Geometry check sheet. Reference: the model listing, model coordinates, mm. Round coordinates to 2 decimals unless told otherwise and drop trailing zeros. Write each loop counter-clockwise with the first axis right and the second up, starting at its lowest first coordinate (ties: lowest second). Pieces come first, ordered by that corner, then holes. Notation, with made-up numbers: M 75,63 L 85,63 A35 ccw 85,101 Z; hole C 51,58.25 d3. An arc over 180 degrees is marked long. Answer as CSV lines item,"result". Start each with the question number.
```python
from build123d import *

# Parameters (mm, degrees)
PROFILE_DEPTH     = 419.1
MITER1_DEPTH      = 422.259210582
MITER1_DEPTH_BACK = 422.259210582
MITER2_DEPTH      = 422.259210582
MITER2_DEPTH_BACK = 422.259210582


with BuildPart() as part:
    # Sketch1 → Profile (new body)
    with BuildSketch(Plane.XY):
        Polygon((-19.05, -38.1), (-4, -38.1), (-4, -30.1), (4, -30.1), (4, -38.1), (19.05, -38.1), (19.05, -23.05), (11.05, -23.05), (11.05, -15.05), (19.05, -15.05), (19.05, 15.05), (11.05, 15.05), (11.05, 23.05), (19.05, 23.05), (19.05, 38.1), (4, 38.1), (4, 30.1), (-4, 30.1), (-4, 38.1), (-19.05, 38.1), (-19.05, 23.05), (-11.05, 23.05), (-11.05, 15.05), (-19.05, 15.05), (-19.05, -15.05), (-11.05, -15.05), (-11.05, -23.05), (-19.05, -23.05), align=None)
    extrude(amount=PROFILE_DEPTH)

    # Sketch2 → Miter1 (cut, two sides: drawn at the far end of the back side and taken through both)
    with BuildSketch(Plane(origin=(0, 0, 0), x_dir=(1, 0, 0), z_dir=(0, 1, 0)).offset(-MITER1_DEPTH_BACK)):
        Polygon((-19.05, -419.1), (25, -342.8), (25, -430), align=None)
    extrude(amount=MITER1_DEPTH + MITER1_DEPTH_BACK, mode=Mode.SUBTRACT)

    # Sketch3 → Miter2 (cut, two sides: drawn at the far end of the back side and taken through both)
    with BuildSketch(Plane(origin=(0, 0, 0), x_dir=(1, 0, 0), z_dir=(0, 1, 0)).offset(-MITER2_DEPTH_BACK)):
        Polygon((-19.05, 0), (25, 10), (25, -25.43), align=None)
    extrude(amount=MITER2_DEPTH + MITER2_DEPTH_BACK, mode=Mode.SUBTRACT)


solid = part.part
```
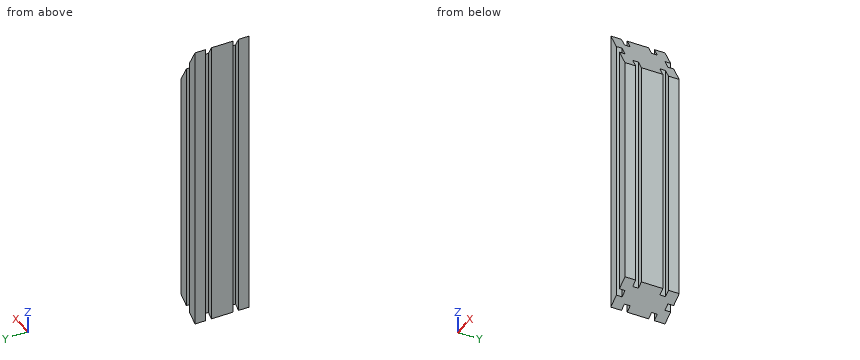
1) Section check B-B, the plane z = 81.5. Record the cut outline in (x, y).
2) Scan lines: line 1 (Y direction, x = -16.5, z = 248); line 2 (X direction, y = 21.5, z = 21.5); line 3 (Y direction, x = 2.5, z = 278). Record each from-to range of solid material in increasing order. Write a range as from..to.
3) Section check A-A, the plane x = 15.5. Record the cut outline in (y, z).
4) Go/stop test with flat-tipped pins: pin 1 (10 mm diameter, centred on x = 1.5, y = 23.5, fed in from -Z); pin 2 (1 mm diameter, centred on x = -2.5, z = 341, fed in from -Y); pin 3 (12 mm diameter, centred on y = -29.5, z = 370, fed in from +X). Record where each tip stops, or that it passes through.
5) Section check D-D, the plane y = 19.5. Record the cut outline in (x, z), plus the area to 3 significant figures.
6) Section check C-C, the plane y = 3. Record the cut outline in (x, z), plus the area to 3 significant figures.
Results:
1,outline,"M -19.05,-38.1 L -4,-38.1 L -4,-30.1 L 4,-30.1 L 4,-38.1 L 19.05,-38.1 L 19.05,-23.05 L 11.05,-23.05 L 11.05,-15.05 L 19.05,-15.05 L 19.05,15.05 L 11.05,15.05 L 11.05,23.05 L 19.05,23.05 L 19.05,38.1 L 4,38.1 L 4,30.1 L -4,30.1 L -4,38.1 L -19.05,38.1 L -19.05,23.05 L -11.05,23.05 L -11.05,15.05 L -19.05,15.05 L -19.05,-15.05 L -11.05,-15.05 L -11.05,-23.05 L -19.05,-23.05 Z"
2,line 1,"y = -38.1..-23.05, -15.05..15.05, 23.05..38.1"
2,line 2,"x = -11.05..11.05"
2,line 3,"y = -30.1..30.1"
3,outline,"M -38.1,19.95 L -23.05,19.95 L -23.05,359.26 L -38.1,359.26 Z; M -15.05,19.95 L 15.05,19.95 L 15.05,359.26 L -15.05,359.26 Z; M 23.05,19.95 L 38.1,19.95 L 38.1,359.26 L 23.05,359.26 Z"
4,pin 1,"stops at z = 8.98"
4,pin 2,"stops at y = -30.1"
4,pin 3,"stops at x = 12.76"
5,outline,"M -11.05,4.62 L 11.05,17.38 L 11.05,366.96 L -11.05,405.24 Z"
5,area,"8,290 mm^2"
6,outline,"M -19.05,0 L 19.05,22 L 19.05,353.11 L -19.05,419.1 Z"
6,area,"14,300 mm^2"
